Design review of the part shown in the three views and the two pictorial views. Dimensions are in mm from the part's minimum x, y and z. A direction names the side the tool comes from. Round coordinates to 2 decimals unless told otherwise and drop trailing zeros. Loops run counter-clockwise (first coordinate to the right, second up) from the corner with the lowest first, then second, coordinate; pieces in that order, holes last. Notation, with made-up numbers: M 77,-27.5 L 126,-27.5 A19 ccw 126,-18.5 Z; hole C 87,79 d9. An arc over 180 degrees is marked long. One line per question, with ' | ' between items. Start each with the question number.
1) For pin 1 Ø4 at (x, y) = (187, 172) entering from -Z; pin 2 Ø15 at (x, z) = (165, 87.5) entering from -Y; pin 3 Ø2 at (x, y) = (86.5, 193) entering from +Z, all flat-tipped, find the tip position at first contact; note any pin that passes through.
2) We need section C-C (y = 149.5). Give the boundary of the cut face in (x, z), and give its area (3 significant figures).
3) We need section B-B (x = 166). Give the boundary of the cut face in (y, z), and give its area (3 significant figures).
4) We need section A-A (z = 46.5). Give the boundary of the cut face in (x, y).
5) Mouldability with a two-part tool opening along X and no side actions: class the marked faces 5, 6, 7 and 8 as pulls with the +X half, pulls with the -X half, needs draft (parallel to the pull), parting line crosses it, or undercut.
6) For probe 1 along X at (y, z) = (113, 65); probe 2 along Y at (x, z) = (114.5, 78); probe 3 along X at (y, z) = (229.5, 113), list the stretches that pass through material, from the lowest coordinate up. Write a range as from..to.
7) For the marked faces 1, 2, 3 and 4, list the 3-axis set-ups (+Z, -Z, +X, -X, +Y, -Y) from which the entire face can be reached by the end or side of a thin tool; tool diameter is ignored.
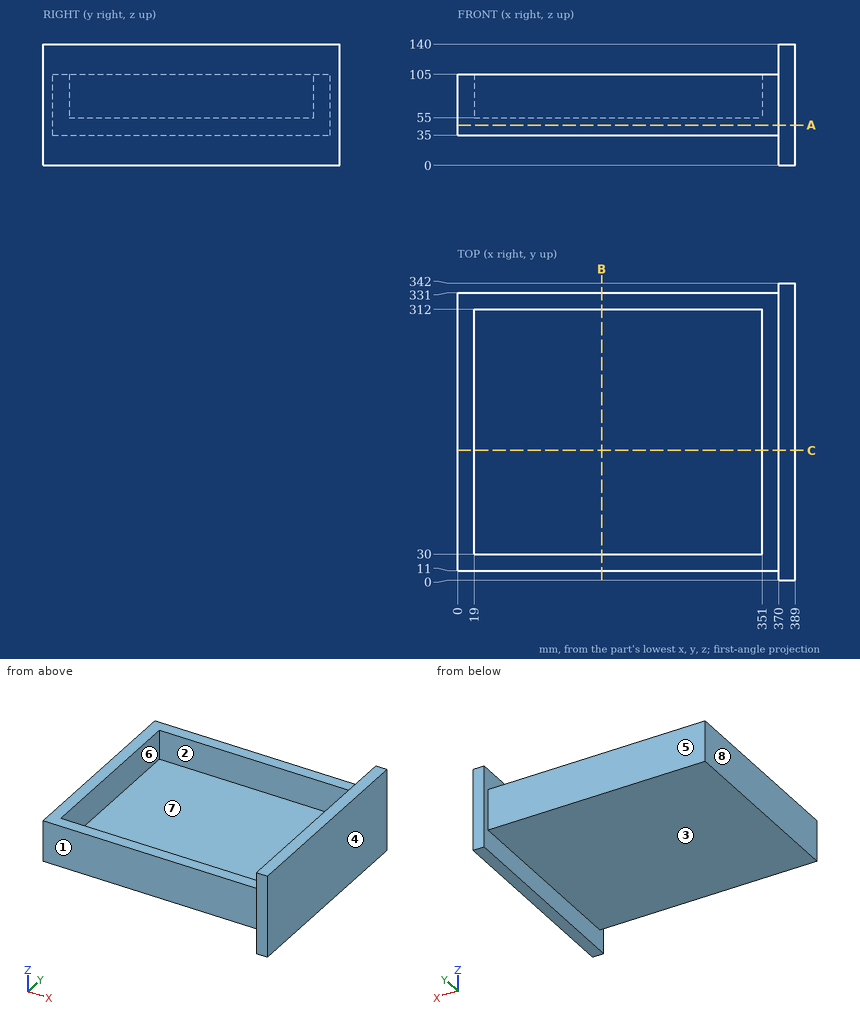
Answers below:
1) pin 1: z = 35 | pin 2: y = 11 | pin 3: z = 55
2) outline: M 0,35 L 370,35 L 370,0 L 389,0 L 389,140 L 370,140 L 370,105 L 351,105 L 351,55 L 19,55 L 19,105 L 0,105 Z | area: 12,000 mm^2
3) outline: M 11,35 L 331,35 L 331,105 L 312,105 L 312,55 L 30,55 L 30,105 L 11,105 Z | area: 8,300 mm^2
4) outline: M 0,11 L 370,11 L 370,0 L 389,0 L 389,342 L 370,342 L 370,331 L 0,331 Z
5) face 5: needs draft | face 6: undercut | face 7: undercut | face 8: pulls with the -X half
6) probe 1: 0..19, 351..389 | probe 2: 11..30, 312..331 | probe 3: 370..389
7) face 1: +Z, -Z, -X, -Y | face 2: +Z | face 3: -Z, -X, +Y, -Y | face 4: +Z, -Z, +X, +Y, -Y
